```python
from build123d import *

# Parameters (mm, degrees)
SKETCH1_W                = 162
SKETCH1_H                = 40
BOSS_EXTRUDE1_DEPTH      = 6
BOSS_EXTRUDE2_START      = -20
SKETCH2_W                = 31.820776168
SKETCH2_H                = 13
BOSS_EXTRUDE2_DEPTH      = 25
CUT_EXTRUDE1_DEPTH       = 97.072888996
BOSS_EXTRUDE3_DEPTH      = 39
BOSS_EXTRUDE3_DEPTH_BACK = 7
SKETCH4_R                = 25
SKETCH5_R                = 12
CUT_EXTRUDE3_DEPTH       = 109.466584762
CUT_EXTRUDE4_DEPTH       = 100.448479124
RIB5_START               = -1
RIB5_DEPTH               = 2


with BuildPart() as part:
    # Sketch1 → Boss-Extrude1 (new body)
    with BuildSketch(Plane.XY):
        Rectangle(SKETCH1_W, SKETCH1_H)
    extrude(amount=-BOSS_EXTRUDE1_DEPTH)

    # Sketch2 → Boss-Extrude2 (add)
    with BuildSketch(Plane(origin=(0, 20, 0), x_dir=(1, 0, 0), z_dir=(0, 1, 0)).offset(BOSS_EXTRUDE2_START)):
        with Locations((0.439513483, 6.5)):
            Rectangle(SKETCH2_W, SKETCH2_H)
    boss_extrude2 = extrude(amount=BOSS_EXTRUDE2_DEPTH)

    # Mirror1: Boss-Extrude2 across plane
    add(boss_extrude2.mirror(Plane.ZX))

    # Sketch3 → Cut-Extrude1 (cut, through all)
    with BuildSketch(Plane(origin=(0, 25, 0), x_dir=(1, 0, 0), z_dir=(0, 1, 0))):
        with BuildLine():
            Line((-12, 0), (12, 0))
            ThreePointArc((12, 0), (0, 12), (-12, 0))
        make_face()
    extrude(amount=-CUT_EXTRUDE1_DEPTH, mode=Mode.SUBTRACT)

    # Sketch4 → Boss-Extrude3 (add, two sides: drawn at the far end of the back side and taken through both)
    with BuildSketch(Plane(origin=(0, 0, -13), x_dir=(-1, 0, 0), z_dir=(0, 0, -1)).offset(-BOSS_EXTRUDE3_DEPTH_BACK)):
        Circle(SKETCH4_R)
    extrude(amount=BOSS_EXTRUDE3_DEPTH + BOSS_EXTRUDE3_DEPTH_BACK)

    # Sketch5 → Cut-Extrude3 (cut, through all)
    with BuildSketch(Plane.XZ.offset(25)):
        Circle(SKETCH5_R)
    extrude(amount=-CUT_EXTRUDE3_DEPTH, mode=Mode.SUBTRACT)

    # Sketch6 → Cut-Extrude4 (cut, through all)
    with BuildSketch(Plane(origin=(0, 0, -52), x_dir=(-1, 0, 0), z_dir=(0, 0, -1))):
        Polygon((0, 13.856406461), (-12, 6.92820323), (-12, -6.92820323), (0, -13.856406461), (12, -6.92820323), (12, 6.92820323), align=None)
    extrude(amount=-CUT_EXTRUDE4_DEPTH, mode=Mode.SUBTRACT)

    # Rib5: read off the stored shape, not the designer's step
    # Rib5 outline → Rib5 (add)
    with BuildSketch(Plane(origin=(0, 0, 0), x_dir=(1, 0, 0), z_dir=(0, 1, 0)).offset(RIB5_START)):
        Polygon((81, 6), (25, 52), (24.979991994, 52), (24.979991994, 6), align=None)
    rib5 = extrude(amount=RIB5_DEPTH)

    # Mirror2: Rib5 across plane
    add(rib5.mirror(Plane(origin=(0, 0, 0), x_dir=(0, 0, 1), z_dir=(1, 0, 0))))


solid = part.part
```
Could you check a few things on this model? Use its own coordinates, in mm. A direction names the side the tool comes from. Coordinates: 2 decimals unless noted, no trailing zeros. Write each loop counter-clockwise with the first axis right and the second up, starting at its lowest first coordinate (ties: lowest second). Pieces come first, ordered by that corner, then holes. Notation, with made-up numbers: (-19.5, 84.5) -> (24.5, 84.5) arc R19 cw to (24.5, 92.5) -> close; hole circle Ø1 at (24.5, -38). An arc over 180 degrees is marked (long way). Write item = value, one per line. Start each with the question number.
(1) I want a section at D-D (z = -9.5). Please give me the cut outline in (x, y).
(2) I want a section at A-A (y = 4). Please give me the cut outline in (x, z), plus the area to 3 significant figures.
(3) We'd pull the mould along Y, two halves only. Please class faces 5 (the face through (46, -1, -24)), 6 (the face through (-49, 11, -6)), 7 (the face through (5.92, 10.44, -32.14)): released by +Y, released by -Y, zero draft, split by the parting line, or undercut.
(4) I want a section at B-B (x = 53). Please give me the cut outline in (y, z), plus the area to 3 significant figures.
(5) I need wall thicknesses on line 1 (X direction, y = -1.5, z = -44); line 2 (Z direction, x = 58.5, y = -6); line 3 (Y direction, x = 68, z = -9). Which ranges of each line are inside material? Lowest first, please. Write a range as [from, to].
(6) Which directions (+Z, -Z, +X, -X, +Y, -Y) give clear straight access to the entire face, cutting with the end or side of a thin tool? Please do faces 1 (the face through (-6.084, 10.344, -32.142)), 2 (the face through (48, 11, -6)), 3 (the face through (-46, -1, -24)), 4 (the face through (-46, 1, -24)).
(7) I want a section at C-C (z = -41). Please give me the cut outline in (x, y), plus the area to 3 significant figures.
(8) Will these pins go through, and if not, where does the flat tip stop? pin 1 (12 mm diameter, centred on x = 57.5, y = 6, fed in from -Z); pin 2 (1.8 mm diameter, centred on x = 43.5, z = -1.5, fed in from -Y); pin 3 (3 mm diameter, centred on x = 47, z = -3, fed in from +Y); pin 4 (4.5 mm diameter, centred on y = 21.5, z = -6.5, fed in from -X).
Result set:
q1.outline = (-76.74, -1) -> (-24.98, -1) arc R25 ccw to (-15.47, -19.64) -> (-15.47, -25) -> (-7.33, -25) -> (-7.33, -9.62) -> (-12, -6.93) -> (-12, 6.93) -> (-7.33, 9.62) -> (-7.33, 25) -> (-15.47, 25) -> (-15.47, 19.64) arc R25 ccw to (-24.98, 1) -> (-76.74, 1) -> close; (7.33, -25) -> (16.35, -25) -> (16.35, -18.91) arc R25 ccw to (24.98, -1) -> (76.74, -1) -> (76.74, 1) -> (24.98, 1) arc R25 ccw to (16.35, 18.91) -> (16.35, 25) -> (7.33, 25) -> (7.33, 9.62) -> (12, 6.93) -> (12, -6.93) -> (7.33, -9.62) -> close
q2.outline = (-81, -6) -> (-24.68, -6) -> (-24.68, -52) -> (-12, -52) -> (-12, 0) -> (-81, 0) -> close; (12, -52) -> (24.68, -52) -> (24.68, -6) -> (81, -6) -> (81, 0) -> (12, 0) -> close
q2.area = 1,990 mm2
q3.face_5 = released by -Y
q3.face_6 = zero draft
q3.face_7 = undercut
q4.outline = (-20, -6) -> (-1, -6) -> (-1, -29) -> (1, -29) -> (1, -6) -> (20, -6) -> (20, 0) -> (-20, 0) -> close
q4.area = 286 mm2
q5.line_1 = [-24.95, -12], [12, 24.95]
q5.line_2 = [-6, 0]
q5.line_3 = [-1, 1]
q6.face_1 = +Z, -Z
q6.face_2 = -Z, +X, +Y
q6.face_3 = -Z, -X, -Y
q6.face_4 = -Z, -X, +Y
q7.outline = (-38.39, -1) -> (-24.98, -1) arc R25 ccw to (24.98, -1) -> (38.39, -1) -> (38.39, 1) -> (24.98, 1) arc R25 ccw to (-24.98, 1) -> (-38.39, 1) -> close; hole (-12, -6.93) -> (0, -13.86) -> (12, -6.93) -> (12, 6.93) -> (0, 13.86) -> (-12, 6.93) -> close
q7.area = 1,520 mm2
q8.pin_1 = -28.03
q8.pin_2 = -20
q8.pin_3 = 20
q8.pin_4 = -81
